For this review, take the finished solid that the model builds, in its own axes (mm). Face numbers are marked on the shaded views. A direction names the side the tool comes from. Give positions to 0.01 mm unless a question says otherwise; leave off trailing zeros. Write each loop counter-clockwise with the first axis right and the second up, starting at its lowest first coordinate (ties: lowest second). Pieces come first, ordered by that corner, then holes.
1) Wall thickness on line 1 along X through (y, z) = (19, 35); line 2 along Z through (x, y) = (12.5, 4.5); line 3 along X through (y, z) = (-66, 20.5): over which ranges is each line inside the solid? List them lowest first.
2) We need section B-B on x = -8.89. Give the boundary of the cut face in (y, z), and give its area (3 significant figures).
3) Draft analysis for pull direction Z (two halves, no side actions). For the marked faces 4, 5, 6 and 7, state which applies: pulls with the +Z half, pulls with the -Z half, needs draft (parallel to the pull), parting line crosses it, or undercut.
4) Machinability: for the marked faces 1, 2 and 3, which of the approach directions +Z, -Z, +X, -X, +Y, -Y give a long, thin tool a straight path to every point of the face, cutting with its end or side? Answer none if there is none.
5) We need section C-C on y = 19.05. Give the boundary of the cut face in (x, z).
6) We need section D-D on x = 4. Give the boundary of the cut face in (y, z), and give its area (3 significant figures).
7) For P1, Ø11.5, axis at x = 4, z = -12.5, coming from the -Y side; P2, Ø3, axis at y = 5, z = -32, coming from the -X side; P3, Ø4.5, axis at x = -8.89, y = 19.05, coming from the -Z side; P4, Ø3, axis at x = -21, y = -86, coming from the -Z side, all flat-tipped, find the tip position at first contact; note any pin that passes through.
8) We need section A-A on z = 0. Give the boundary of the cut face in (x, y), and give its area (3 significant figures).
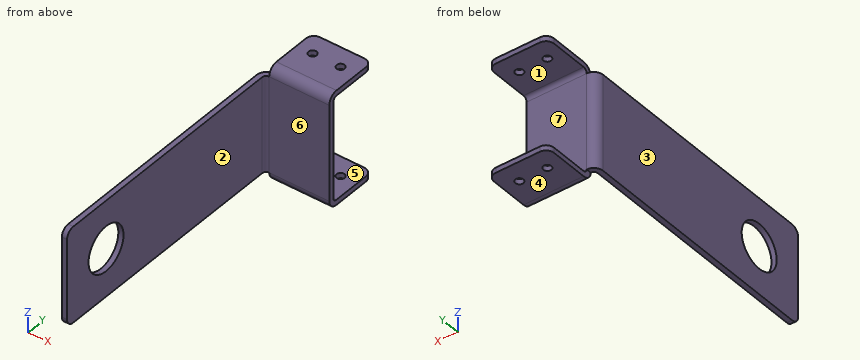
from build123d import *

# Parameters (mm, degrees)
SKETCH1_W               = 38.1
SKETCH1_H               = 60.96
BASE_FLANGE1_DEPTH      = 3.302
EDGE_FLANGE1_DEPTH      = 38.1
EDGE_FLANGE1_BEND_DEPTH = 38.1
EDGE_FLANGE2_DEPTH      = 60.96
SKETCH17_R              = 14.28115
CUT_EXTRUDE1_DEPTH      = 175.665958469
F_1_4_20_TAPPED_HOLE1_D = 5.1054
FILLET1_R               = 5.08


# Sheet-metal steps are written as plain solids
with BuildPart() as part:
    # Sketch1 → Base-Flange1 (new body)
    with BuildSketch(Plane(origin=(0, 0, 0), x_dir=(1, 0, 0), z_dir=(0, 1, 0))):
        Rectangle(SKETCH1_W, SKETCH1_H)
    extrude(amount=-BASE_FLANGE1_DEPTH)

    # Edge-Flange1 section (across the edge) → Edge-Flange1 (add)
    with BuildSketch(Plane(origin=(-19.05, 0, 33.02), x_dir=(0, 0, -1), z_dir=(1, 0, 0))):
        with BuildLine():
            Line((-3.302, 2.54), (-3.302, 31.75))
            Line((-3.302, 31.75), (0, 31.75))
            Line((0, 31.75), (0, 2.54))
            ThreePointArc((0, 2.54), (0.743948776, 0.743948776), (2.54, 0))
            Line((2.54, 0), (2.54, -3.302))
            ThreePointArc((2.54, -3.302), (-1.590917816, -1.590917816), (-3.302, 2.54))
        make_face()
    extrude(amount=EDGE_FLANGE1_DEPTH)

    # Edge-Flange1 section 2 (across the edge) → Edge-Flange1 bend (add)
    with BuildSketch(Plane(origin=(19.05, 0, -33.02), x_dir=(0, 0, 1), z_dir=(-1, 0, 0))):
        with BuildLine():
            Line((-3.302, 2.54), (-3.302, 31.75))
            Line((-3.302, 31.75), (0, 31.75))
            Line((0, 31.75), (0, 2.54))
            ThreePointArc((0, 2.54), (0.743948776, 0.743948776), (2.54, 0))
            Line((2.54, 0), (2.54, -3.302))
            ThreePointArc((2.54, -3.302), (-1.590917816, -1.590917816), (-3.302, 2.54))
        make_face()
    extrude(amount=EDGE_FLANGE1_BEND_DEPTH)

    # Edge-Flange2 section (across the edge) → Edge-Flange2 (add)
    with BuildSketch(Plane(origin=(-21.59, -3.302, 30.48), x_dir=(1, 0, 0), z_dir=(0, 0, -1))):
        with BuildLine():
            Line((-3.302, 2.54), (-3.302, 161.798))
            Line((-3.302, 161.798), (0, 161.798))
            Line((0, 161.798), (0, 2.54))
            ThreePointArc((0, 2.54), (0.743948776, 0.743948776), (2.54, 0))
            Line((2.54, 0), (2.54, -3.302))
            ThreePointArc((2.54, -3.302), (-1.590917816, -1.590917816), (-3.302, 2.54))
        make_face()
    extrude(amount=EDGE_FLANGE2_DEPTH)

    # Sketch17 → Cut-Extrude1 (cut, through all)
    with BuildSketch(Plane.ZY.offset(24.892)):
        with Locations(Location((0, -133.2738, 0), (0, 0, 270))):
            Circle(SKETCH17_R)
    extrude(amount=-CUT_EXTRUDE1_DEPTH, mode=Mode.SUBTRACT)

    # 1/4-20 Tapped Hole1 (through all)
    with Locations(Plane.XY.offset(36.322)):
        with Locations((8.89, 19.05), (-8.89, 19.05)):
            Hole(F_1_4_20_TAPPED_HOLE1_D / 2)

    # Fillet1
    fillet1_edges = [part.edges().sort_by_distance(p)[0] for p in [
        (-19.05, 31.75, 34.671),
        (19.05, 31.75, 34.671),
        (19.05, 31.75, -34.671),
        (-19.05, 31.75, -34.671),
        (-23.241, -165.1, 30.48),
        (-23.241, -165.1, -30.48),
    ]]
    fillet(fillet1_edges, radius=FILLET1_R)


solid = part.part
Results list:
1. line 1: x = -19.05 to -11.44, -6.34 to 6.34, 11.44 to 19.05
1. line 2: z = -36.32 to -33.02, 33.02 to 36.32
1. line 3: x = -24.89 to -21.59
2. outline: (-3.3, -30.48) arc R5.84 ccw to (2.54, -36.32) - (16.5, -36.32) - (16.5, -33.02) - (2.54, -33.02) arc R2.54 cw to (0, -30.48) - (0, 30.48) arc R2.54 cw to (2.54, 33.02) - (16.5, 33.02) - (16.5, 36.32) - (2.54, 36.32) arc R5.84 ccw to (-3.3, 30.48) - close; (21.6, -36.32) - (31.75, -36.32) - (31.75, -33.02) - (21.6, -33.02) - close; (21.6, 33.02) - (31.75, 33.02) - (31.75, 36.32) - (21.6, 36.32) - close
2. area: 404 mm2
3. face 4: pulls with the -Z half
3. face 5: undercut
3. face 6: needs draft
3. face 7: undercut
4. face 1: +X, -X, +Y
4. face 2: +Z, -Z, +X, -Y
4. face 3: +Z, -Z, -X, +Y, -Y
5. outline: (-19.05, -36.32) - (-11.44, -36.32) - (-11.44, -33.02) - (-19.05, -33.02) - close; (-19.05, 33.02) - (-11.44, 33.02) - (-11.44, 36.32) - (-19.05, 36.32) - close; (-6.34, -36.32) - (6.34, -36.32) - (6.34, -33.02) - (-6.34, -33.02) - close; (-6.34, 33.02) - (6.34, 33.02) - (6.34, 36.32) - (-6.34, 36.32) - close; (11.44, -36.32) - (19.05, -36.32) - (19.05, -33.02) - (11.44, -33.02) - close; (11.44, 33.02) - (19.05, 33.02) - (19.05, 36.32) - (11.44, 36.32) - close
6. outline: (-3.3, -30.48) arc R5.84 ccw to (2.54, -36.32) - (31.75, -36.32) - (31.75, -33.02) - (2.54, -33.02) arc R2.54 cw to (0, -30.48) - (0, 30.48) arc R2.54 cw to (2.54, 33.02) - (31.75, 33.02) - (31.75, 36.32) - (2.54, 36.32) arc R5.84 ccw to (-3.3, 30.48) - close
6. area: 438 mm2
7. P1: stops at y = -3.3
7. P2: stops at x = -19.05
7. P3: passes through
7. P4: stops at z = -30.48
8. outline: (-24.89, -165.1) - (-21.59, -165.1) - (-21.59, -147.55) - (-24.89, -147.55) - close; (-24.89, -118.99) - (-21.59, -118.99) - (-21.59, -5.84) arc R2.54 cw to (-19.05, -3.3) - (19.05, -3.3) - (19.05, 0) - (-19.05, 0) arc R5.84 ccw to (-24.89, -5.84) - close
8. area: 579 mm2
